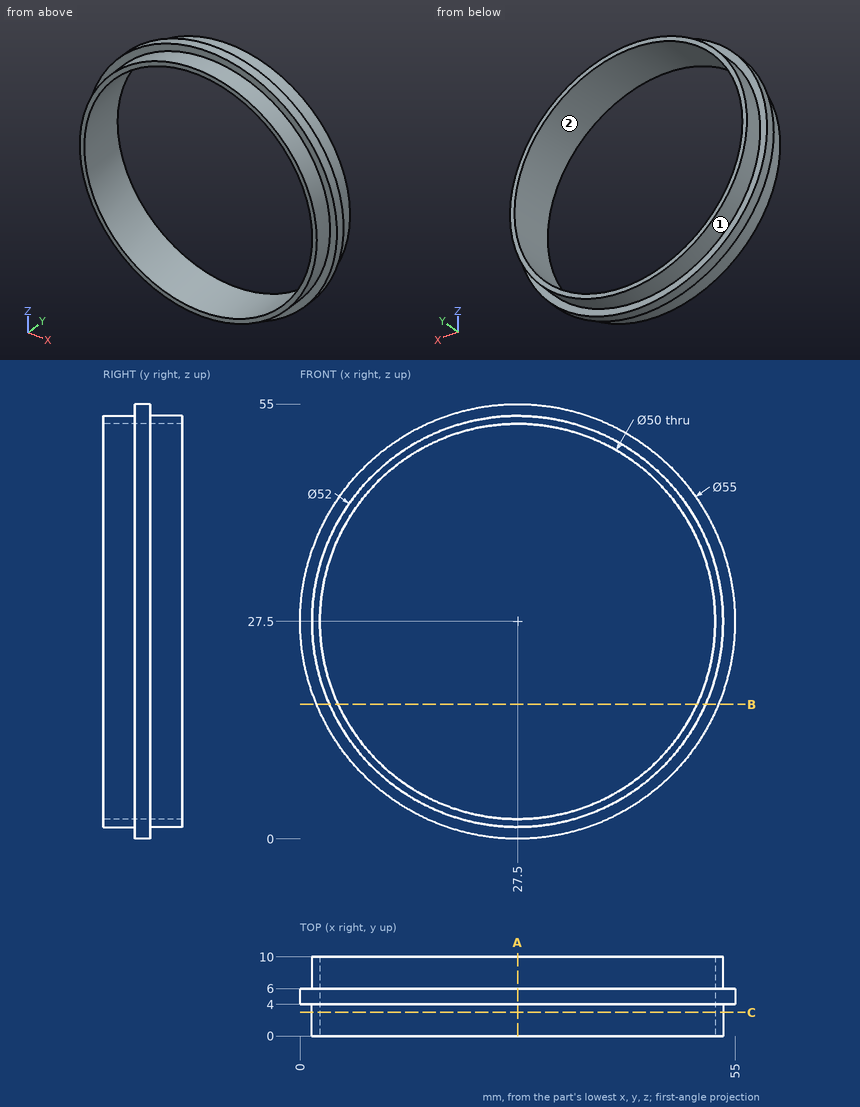
Part print with two shaded views. Sizes in mm from the minimum x, y, z corner. Give positions to 0.01 mm unless a question says otherwise; leave off trailing zeros. Loops run counter-clockwise (first coordinate to the right, second up) from the corner with the lowest first, then second, coordinate; pieces in that order, holes last. Notation, with made-up numbers: (-25.5, 13) - (20.5, 13) arc R9 ccw to (20.5, 18) - close; hole circle Ø1 at (-6, 89). An arc over 180 degrees is marked (long way). Put each result on its own line as item: value.
Q1. Slice it at A-A (x = 27.5). Give the cut face in (y, z).
Filled in:
outline: (0, 1.5) - (4, 1.5) - (4, 0) - (6, 0) - (6, 1.5) - (10, 1.5) - (10, 2.5) - (0, 2.5) - close; (0, 52.5) - (10, 52.5) - (10, 53.5) - (6, 53.5) - (6, 55) - (4, 55) - (4, 53.5) - (0, 53.5) - close
Q2. Probe line 1 along Z through (x, y) = (27.5, 7.5); line 2 along Z through (x, y) = (27.5, 5). List the from-to ranges inside material, lowest first.
Filled in:
line 1: z = 1.5 to 2.5, 52.5 to 53.5
line 2: z = 0 to 2.5, 52.5 to 55
Q3. Slice it at B-B (z = 17). Give the cut face in (x, y), plus the area to 3 significant figures.
Filled in:
outline: (2.08, 4) - (3.71, 4) - (3.71, 0) - (4.81, 0) - (4.81, 10) - (3.71, 10) - (3.71, 6) - (2.08, 6) - close; (50.19, 0) - (51.29, 0) - (51.29, 4) - (52.92, 4) - (52.92, 6) - (51.29, 6) - (51.29, 10) - (50.19, 10) - close
area: 28.5 mm²
Q4. Slice it at C-C (y = 3). Give the cut face in (x, z).
Filled in:
outline: circle Ø52 at (27.5, 27.5); hole circle Ø50 at (27.5, 27.5)
Q5. Mould opens along X. For the marked faces 1 and 2 say: pulls with the +X half, pulls with the -X half, needs draft (parallel to the pull), parting line crosses it, or undercut.
Filled in:
face 1: parting line crosses it
face 2: undercut
Q6. Flat gauge pins, fed straight in: pin 1 (6 mm diameter, centred on x = 45, z = 44.5, fed in from -Y); pin 2 (4 mm diameter, centred on x = 41, y = 9, fed in from -Z); pin 3 (2 mm diameter, centred on y = 3.5, z = 25, fed in from -X). Where does each tip first touch, or does it go through?
Filled in:
pin 1: stops at y = 0
pin 2: stops at z = 4.18
pin 3: stops at x = 0.05
